Part model, mm, in its own coordinate system. Coordinates: 2 decimals unless noted, no trailing zeros. Write each loop counter-clockwise with the first axis right and the second up, starting at its lowest first coordinate (ties: lowest second). Pieces come first, ordered by that corner, then holes. Notation, with made-up numbers: (18, 14) -> (57, 14) arc R26 ccw to (57, 31) -> close; hole circle Ø5 at (30, 78). An arc over 180 degrees is marked (long way). Write item = value, one per line.
Autodesk Inventor part; units mm, degrees
ref_plane "YZ Plane" through (0, 0, 0) normal (1, 0, 0) x (0, 1, 0)
ref_plane "XZ Plane" through (0, 0, 0) normal (0, 1, 0) x (-1, 0, 0)
ref_plane "XY Plane" through (0, 0, 0) normal (0, 0, 1) x (1, 0, 0)
sketch "Sketch1" plane through (0, 0, 0) normal (0, 0, 1) x (1, 0, 0)
  line L0 (-203.2, -6.35) -> (-203.2, 584.2)
  arc A0 (-184.15, 603.25) -> (-203.2, 584.2) centre (-184.15, 584.2) ccw
  line L1 (-184.15, -6.35) -> (-184.15, 565.15)
  arc A1 (-165.1, 584.2) -> (-184.15, 565.15) centre (-165.1, 565.15) ccw
  line L2 (-203.2, -6.35) -> (-184.15, -6.35)
  line L3 (203.2, -6.35) -> (203.2, 584.2)
  arc A2 (203.2, 584.2) -> (184.15, 603.25) centre (184.15, 584.2) ccw
  line L4 (184.15, -6.35) -> (184.15, 565.15)
  arc A3 (184.15, 565.15) -> (165.1, 584.2) centre (165.1, 565.15) ccw
  line L5 (203.2, -6.35) -> (184.15, -6.35)
  line L6 (165.1, 584.2) -> (-165.1, 584.2)
  line L7 (-184.15, 603.25) -> (184.15, 603.25)
  point P0 (0, 0)
  dimension "d7" = 406.4
  dimension "d31" = 609.6
  dimension "d32" = 609.6
  dimension "d33" = 19.05
extrude "Extrusion1" add sketch "Sketch1" along normal mid plane 19.05
fillet "Fillet1" radius 9.525 20 edges at (178.5704, 578.6204, 9.525) (0, 584.2, 9.525) (-178.5704, 578.6204, 9.525) (-184.15, 279.4, 9.525) (184.15, 279.4, 9.525) (197.6204, 597.6704, 9.525) (0, 603.25, 9.525) (-197.6204, 597.6704, 9.525) (-203.2, 288.925, 9.525) (203.2, 288.925, 9.525) (197.6204, 597.6704, -9.525) (0, 603.25, -9.525) (-197.6204, 597.6704, -9.525) (-203.2, 288.925, -9.525) (203.2, 288.925, -9.525) (178.5704, 578.6204, -9.525) (0, 584.2, -9.525) (-178.5704, 578.6204, -9.525) (-184.15, 279.4, -9.525) (184.15, 279.4, -9.525)
sketch "Sketch2" plane through (0, 0, 0) normal (0, 0, 1) x (1, 0, 0)
  line L0 (203.2, 584.2) -> (203.2, -6.35)
  line L1 (203.2, 247.65) -> (193.675, 247.65)
  line L2 (193.675, 247.65) -> (193.675, 273.05)
  line L3 (193.675, 273.05) -> (203.2, 273.05)
  line L4 (203.2, 273.05) -> (203.2, 247.65)
  line L5 (203.2, -6.35) -> (184.15, -6.35)
  line L6 (-203.2, -6.35) -> (-203.2, 584.2)
  line L7 (-203.2, 273.05) -> (-193.675, 273.05)
  line L8 (-193.675, 273.05) -> (-193.675, 247.65)
  line L9 (-193.675, 247.65) -> (-203.2, 247.65)
  line L10 (-203.2, 247.65) -> (-203.2, 273.05)
  line L11 (-184.15, -6.35) -> (-203.2, -6.35)
  point P0 (0, 0)
  dimension "d13" = 254
  dimension "d14" = 25.4
  dimension "d15" = 9.525
  dimension "d16" = 25.4
  dimension "d17" = 254
  dimension "d34" = 387.35
extrude "Extrusion2" add sketch "Sketch2" along normal blind 44.45
sketch "Sketch3" plane through (203.2, 247.65, 0) normal (1, 0, 0) x (0, 0, -1)
  line L0 (0, 25.4) -> (-44.45, 25.4)
  line L1 (-44.45, 0) -> (-44.45, 25.4)
  point P0 (0, -247.65)
  point P1 (-25.4, 12.7)
  dimension "d20" = 12.7
  dimension "d21" = 19.05
hole "Hole1" at (203.2, 260.35, 25.4) direction (-1, 0, 0) diameter 12.7 end through all
properties part number "support"
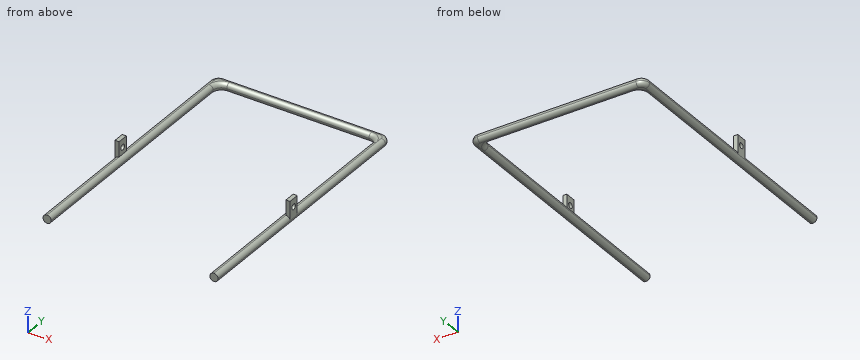
Q1. Pin check, flat tips, straight feed: pin 1 (7.5 mm diameter, centred on x = 199, z = 24, fed in from -Y); pin 2 (8 mm diameter, centred on x = -11.5, z = -1, fed in from -Y); pin 3 (8 mm diameter, centred on y = 410.5, z = 5.5, fed in from -X). Stop position of each tip, or through.
Model answer:
pin_1 = 247.65
pin_2 = 584.2
pin_3 = -203.08
Q2. Probe line 1 (X direction, y = 170.5, z = -1); line 2 (Y direction, x = -196.25, z = 25.4); line 3 (X direction, y = 185, z = -1.5). List the from-to ranges inside material, lowest first. Write a range as from..to.
Model answer:
line_1 = -203.15..-184.2, 184.2..203.15
line_2 = 247.65..254, 266.7..273.05
line_3 = -203.08..-184.27, 184.27..203.08
Q3. Saw through at A-A on y = 260.35. Count the separate pieces of the cut face and the enclosed holes in it, and give its area (3 significant figures).
Model answer:
separate_pieces = 4
enclosed_holes = 0
area = 1,030 mm²
Q4. Saw through at B-B on z = 25.4. Give the cut face in (x, y) (3 decimals).
Model answer:
outline = (-203.2, 247.65) -> (-193.675, 247.65) -> (-193.675, 254) -> (-203.2, 254) -> close; (-203.2, 266.7) -> (-193.675, 266.7) -> (-193.675, 273.05) -> (-203.2, 273.05) -> close; (193.675, 247.65) -> (203.2, 247.65) -> (203.2, 254) -> (193.675, 254) -> close; (193.675, 266.7) -> (203.2, 266.7) -> (203.2, 273.05) -> (193.675, 273.05) -> close
